Input: dimensioned drawing with shaded views. Units: mm. Origin: part minimum x, y, z. Round coordinates to 2 decimals unless told otherwise and drop trailing zeros. Loops run counter-clockwise (first coordinate to the right, second up) from the corner with the lowest first, then second, coordinate; pieces in that order, holes last. Notation, with made-up numbers: M 23.5,62 L 69.5,62 A19 cw 69.5,82 Z; hole C 68.25,53 d1. An arc over 180 degrees is marked long. Answer as a JSON object with one key per item and string values.
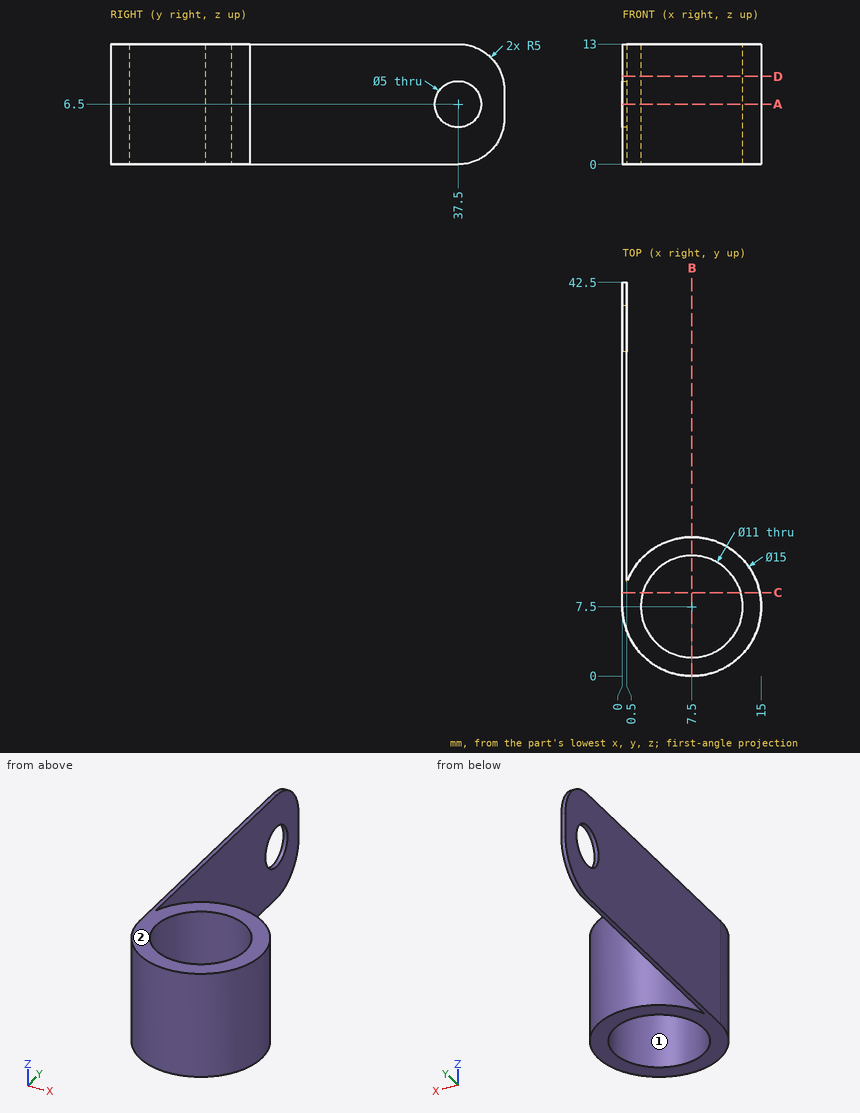
Item 1: Section A-A on z = 6.5. Return the cut outline in (x, y), then the cut area to 3 significant figures.
Answer sheet:
{"outline": "M 0,7.5 A7.5 ccw long 0.5,10.19 L 0.5,35 L 0,35 Z; M 0,40 L 0.5,40 L 0.5,42.5 L 0,42.5 Z; hole C 7.5,7.5 d11", "area": "95.8 mm²"}
Item 2: Section D-D on z = 9.5. Return the cut outline in (x, y).
Answer sheet:
{"outline": "M 0,7.5 A7.5 ccw long 0.5,10.19 L 0.5,42.27 L 0,42.27 Z; hole C 7.5,7.5 d11"}
Item 3: Line query: probe 1 along Y at (x, z) = (7.5, 6); probe 2 along X at (y, z) = (29.5, 0.75); probe 3 along Y at (x, z) = (9, 5.5). Output: solid intervals per line, ascending. Write a range as from..to.
Answer sheet:
{"probe 1": "y = 0..2, 13..15", "probe 2": "x = 0..0.5", "probe 3": "y = 0.15..2.21, 12.79..14.85"}
Item 4: Contact query for flat-ended pins moving along their axis: pin 1 Ø5 at (x, z) = (13, 2.5) entering from +Y; pin 2 Ø2 at (y, z) = (18.5, 8) entering from +X; pin 3 Ø1.5 at (x, z) = (4.5, 10) entering from -Y. Output: stop coordinate, or through.
Answer sheet:
{"pin 1": "stops at y = 14.37", "pin 2": "stops at x = 0.5", "pin 3": "stops at y = 0.35"}
Item 5: Section B-B on x = 7.5. Return the cut outline in (y, z).
Answer sheet:
{"outline": "M 0,0 L 2,0 L 2,13 L 0,13 Z; M 13,0 L 15,0 L 15,13 L 13,13 Z"}
Item 6: Pull-direction query (Y, two-part tool) for the marked faces 1 and 2; classes: pulls with the +Y half, pulls with the -Y half, needs draft (parallel to the pull), parting line crosses it, or undercut.
Answer sheet:
{"face 1": "undercut", "face 2": "needs draft"}
Item 7: Section C-C on y = 9. Return the cut outline in (x, z).
Answer sheet:
{"outline": "M 0,0 L 2.21,0 L 2.21,13 L 0,13 Z; M 12.79,0 L 14.85,0 L 14.85,13 L 12.79,13 Z"}
